Here's how the part is built. I have some questions about the finished solid (model axes, mm). A direction names the side the tool comes from. Coordinates: 2 decimals unless noted, no trailing zeros. Write each loop counter-clockwise with the first axis right and the second up, starting at its lowest first coordinate (ties: lowest second). Pieces come first, ordered by that corner, then holes.
from build123d import *

# Parameters (mm, degrees)
F0_W     = 140
F0_H     = 35
F1_DEPTH = 15
F3_DEPTH = 140


with BuildPart() as f1:
    # F0 (on Front) → F1 (new body)
    with BuildSketch(Plane.XZ):
        Rectangle(F0_W, F0_H)
    extrude(amount=F1_DEPTH)

    # F2 (on face) → F3 (cut, through all)
    with BuildSketch(Plane.YZ.offset(70)):
        Polygon((-15, 14.5), (-15, -17.5), (-12, -17.5), (-12, 6.5), (-11, 6.5), (-11, 14.5), align=None)
    extrude(amount=-F3_DEPTH, mode=Mode.SUBTRACT)


solid = f1.part
1. I want a section at B-B (z = 11.5). List the corners of the cut face in (x, y) for me.
2. For pin 1 Ø1.2 at (x, y) = (-22, -13) entering from -Z; pin 2 Ø9 at (x, z) = (4, 9) entering from -Y, each with a flat end and sliding along its axis, tell me the tip position at first contact or that it passes through.
3. If I drill on line 1 (Z direction, x = -51.5, y = -11.5); line 2 (Z direction, x = 32.5, y = -14); line 3 (Y direction, x = -27.5, z = -14), over which ranges is the centre line in solid material (lowest first)?
4. I want a section at A-A (x = 57.5). List the corners of the cut face in (y, z) for me.
5. On a 3-axis mill with a long thin cutter (end or side, diameter ignored), from which of +Z, -Z, +X, -X, +Y, -Y can I reach the whole of each face in a straight line? I mean faces 1 (the face through (1, -13, 14.5)), 2 (the face through (1, -12, -6)), 3 (the face through (70, -6, 0)). Say none if no direction works.
6. I want a section at C-C (z = 0). List the corners of the cut face in (x, y) for me, then the cut area to 3 significant figures.
Response values:
1. outline: (-70, -11) - (70, -11) - (70, 0) - (-70, 0) - close
2. pin 1: stops at z = 14.5
2. pin 2: stops at y = -12
3. line 1: z = -17.5 to 6.5, 14.5 to 17.5
3. line 2: z = 14.5 to 17.5
3. line 3: y = -12 to 0
4. outline: (-15, 14.5) - (-11, 14.5) - (-11, 6.5) - (-12, 6.5) - (-12, -17.5) - (0, -17.5) - (0, 17.5) - (-15, 17.5) - close
5. face 1: +X, -X, -Y
5. face 2: -Z, +X, -X, -Y
5. face 3: +Z, -Z, +X, +Y, -Y
6. outline: (-70, -12) - (70, -12) - (70, 0) - (-70, 0) - close
6. area: 1,680 mm2
